Build history of the part. All positions in model axes, mm. A direction names the side the tool comes from. Round coordinates to 2 decimals unless told otherwise and drop trailing zeros. Loops run counter-clockwise (first coordinate to the right, second up) from the corner with the lowest first, then second, coordinate; pieces in that order, holes last. Notation, with made-up numbers: (-29, 27.5) - (21, 27.5) arc R19 ccw to (21, 63.5) - close; hole circle Ø5 at (-20.5, 25). An arc over 180 degrees is marked (long way). Use a Markdown table: item, result.
from build123d import *

# Parameters (mm, degrees)
SKETCH1_R           = 18.5
BOSS_EXTRUDE1_DEPTH = 53
SKETCH2_R           = 6
SKETCH2_R_2         = 3
BOSS_EXTRUDE2_DEPTH = 5
SKETCH2_3_R         = 3
BOSS_EXTRUDE3_DEPTH = 20
SKETCH4_W           = 9.457424045
SKETCH4_H           = 2.618978966
CUT_EXTRUDE1_DEPTH  = 14
CIRPATTERN1_COUNT   = 6


with BuildPart() as part:
    # Sketch1 → Boss-Extrude1 (new body)
    with BuildSketch(Plane(origin=(0, 0, 0), x_dir=(1, 0, 0), z_dir=(0, 1, 0))):
        with Locations(Location((0, 0, 0), (0, 0, 270))):
            Circle(SKETCH1_R)
    extrude(amount=BOSS_EXTRUDE1_DEPTH)

    # Sketch2 → Boss-Extrude2 (add)
    with BuildSketch(Plane(origin=(0, 53, 0), x_dir=(1, 0, 0), z_dir=(0, 1, 0))):
        with Locations(Location((0, 7, 0), (0, 0, 270))):
            Circle(SKETCH2_R)
        with Locations(Location((0, 7, 0), (0, 0, 270))):
            Circle(SKETCH2_R_2, mode=Mode.SUBTRACT)
    extrude(amount=BOSS_EXTRUDE2_DEPTH)

    # Sketch2_3 → Boss-Extrude3 (add)
    with BuildSketch(Plane(origin=(0, 53, 0), x_dir=(1, 0, 0), z_dir=(0, 1, 0))):
        with Locations(Location((0, 7, 0), (0, 0, 270))):
            Circle(SKETCH2_3_R)
    extrude(amount=BOSS_EXTRUDE3_DEPTH)

    # Sketch4 → Cut-Extrude1 (cut)
    with BuildSketch(Plane(origin=(0, 73, 0), x_dir=(1, 0, 0), z_dir=(0, 1, 0))):
        with Locations((0.928983292, 10.809489483)):
            Rectangle(SKETCH4_W, SKETCH4_H)
    extrude(amount=-CUT_EXTRUDE1_DEPTH, mode=Mode.SUBTRACT)

    # Sketch7 → M3x0.5 Tapped Hole1 (revolve, cut)
    with BuildSketch(Plane(origin=(7.75, 53, -13.423393759), x_dir=(0, 0, 1), z_dir=(1, 0, 0))):
        Polygon((0, 0), (0, 8.751075774), (1.25, 8), (1.25, 0.316351312), (1.525, 0), align=None)
    m3x0_5_tapped_hole1 = revolve(axis=Axis((7.75, 59.35, -13.423393759), (0, -1, 0)), mode=Mode.SUBTRACT)

    # CirPattern1: M3x0.5 Tapped Hole1 ×6 about axis
    cirpattern1_axis = Axis((0, 0, 0), (0, 1, 0))
    for i in range(1, CIRPATTERN1_COUNT):
        add(m3x0_5_tapped_hole1.rotate(cirpattern1_axis, i * 360 / CIRPATTERN1_COUNT), mode=Mode.SUBTRACT)


solid = part.part
Q1. Cut at A-A, the plane x = -4. List the corners of the cut face in (y, z).
Results found:
| item | result |
|---|---|
| outline | (0, -18.06) - (53, -18.06) - (53, -11.47) - (58, -11.47) - (58, -2.53) - (53, -2.53) - (53, 18.06) - (0, 18.06) - close |
Q2. Cut at B-B, the plane z = -6.5. List the corners of the cut face in (x, y).
Results found:
| item | result |
|---|---|
| outline | (-17.32, 0) - (17.32, 0) - (17.32, 53) - (5.98, 53) - (5.98, 58) - (2.96, 58) - (2.96, 73) - (-2.96, 73) - (-2.96, 58) - (-5.98, 58) - (-5.98, 53) - (-17.32, 53) - close |
Q3. Cut at C-C, the plane y = 27. List the corners of the cut face in (x, z), plus the area to 3 significant figures.
Results found:
| item | result |
|---|---|
| outline | circle Ø37 at (0, 0) |
| area | 1,080 mm2 |
Q4. Pull direction Z, two halves, no side cores. Call faces 4 (the face through (7.6, 44.38, -13.58)), 5 (the face through (4.06, 55.46, -11.42)), 6 (the face through (-1, 58, -10)), 7 (the face through (-8.86, 48.9, -14)): pulls with the +Z half, pulls with the -Z half, needs draft (parallel to the pull), parting line crosses it, or undercut.
Results found:
| item | result |
|---|---|
| face 4 | undercut |
| face 5 | parting line crosses it |
| face 6 | needs draft |
| face 7 | undercut |
Q5. Which spindle directions (+Z, -Z, +X, -X, +Y, -Y) get a long thin tool onto all of the face, cutting with end or side? Do faces 1 (the face through (-8.97, 48.9, 13.69)), 2 (the face through (0, 73, -7)), 3 (the face through (0, 66, -9.5)). Say none if no direction does.
Results found:
| item | result |
|---|---|
| face 1 | +Y |
| face 2 | +Z, -Z, +X, -X, +Y |
| face 3 | -Z, +X, -X, +Y |
Q6. Cut at D-D, the plane x = 0. List the corners of the cut face in (y, z).
Results found:
| item | result |
|---|---|
| outline | (0, -18.5) - (53, -18.5) - (53, -13) - (58, -13) - (58, -10) - (59, -10) - (59, -9.5) - (73, -9.5) - (73, -4) - (58, -4) - (58, -1) - (53, -1) - (53, 18.5) - (0, 18.5) - close |
Q7. Probe line 1 (Y direction, x = -6, z = 0); line 2 (Z direction, x = 7, y = 49); line 3 (X direction, y = 51.5, z = 12.5). List the from-to ranges inside material, lowest first.
Results found:
| item | result |
|---|---|
| line 1 | y = 0 to 53 |
| line 2 | z = -17.12 to -14.42, -12.42 to 12.42, 14.42 to 17.12 |
| line 3 | x = -13.64 to -8.59, -6.91 to 6.91, 8.59 to 13.64 |
Q8. Drop flat-ended pins along their axis: pin 1 (5 mm diameter, centred on x = 3.5, y = 23, fed in from -Z); pin 2 (1 mm diameter, centred on x = -8, y = 45.5, fed in from -Z); pin 3 (3.5 mm diameter, centred on x = 0, y = 63, fed in from -Z). Give the stop position or say it passes through.
Results found:
| item | result |
|---|---|
| pin 1 | stops at z = -18.47 |
| pin 2 | stops at z = -16.91 |
| pin 3 | stops at z = -9.5 |
